Here's how the part is built. I have some questions about the finished solid (model axes, mm). Coordinates: 2 decimals unless noted, no trailing zeros. Write each loop counter-clockwise with the first axis right and the second up, starting at its lowest first coordinate (ties: lowest second). Pieces come first, ordered by that corner, then holes. Notation, with made-up numbers: (27, -0.75) -> (50, -0.75) arc R16 ccw to (50, 30.25) -> close; hole circle Ø8 at (6, 37). An arc over 180 degrees is marked (long way). Use a Markdown table: item, result. Add a question column.
Item 1: Imagine slicing it at B-B, the plane x = 0. Write out the boundary of the cut face in (y, z).
Item 2: Will these pins go through, and if not, where does the flat tip stop? pin 1 Ø4 at (x, y) = (1.5, -10.5) entering from -Z; pin 2 Ø6 at (y, z) = (3.5, 3) entering from -X; pin 3 Ø4 at (y, z) = (-18.5, 3) entering from -X; pin 4 Ø2 at (x, z) = (-4, 2.5) entering from +Y.
Item 3: Imagine slicing it at A-A, the plane z = 0. Write out the boundary of the cut face in (x, y).
Item 4: Imagine slicing it at D-D, the plane y = -25.5. Write out the boundary of the cut face in (x, z).
Item 5: Imagine slicing it at C-C, the plane y = 7. Write out the boundary of the cut face in (x, z), and give its area (3 significant figures).
Item 6: If I drill on line 1 along Z through (x, y) = (0.25, -85.5); line 2 along Z through (x, y) = (1.75, -30.5); line 3 along Y through (x, z) = (-4.25, -1.5), over which ranges is the centre line in solid material (lowest first)? Write a range as from..to.
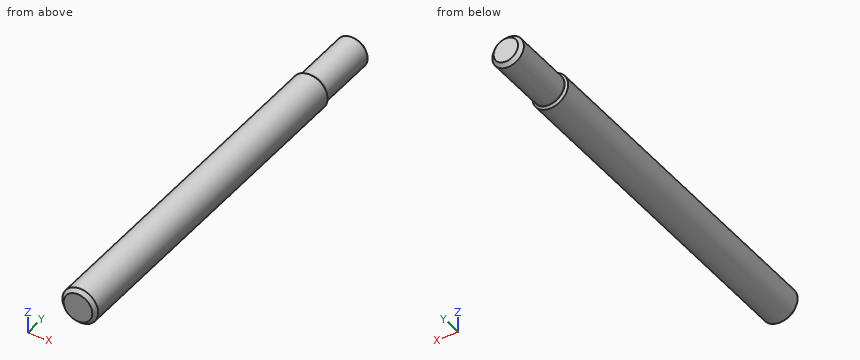
```python
from build123d import *

# Parameters (mm, degrees)
F0_R        = 5
F1_DEPTH    = 100
F2_R        = 4.4
F3_DEPTH    = 18
F4_S5_R     = 4.4
F4_T6_DEPTH = 9
F5_SIZE     = 1


# Not quite as in the source:
# - a fillet or chamfer that OpenCascade refuses, or shapes differently, is made with other operations: its cross-section is extruded or revolved along the edge and cut away or added


with BuildPart() as f1:
    # F0 (on Front) → F1 (new body)
    with BuildSketch(Plane.XZ):
        Circle(F0_R)
    extrude(amount=F1_DEPTH)

    # F2 (on face) → F3 (join)
    with BuildSketch(Plane(origin=(0, 0, 0), x_dir=(-1, 0, 0), z_dir=(0, 1, 0))):
        Circle(F2_R)
    extrude(amount=F3_DEPTH)

    # F4: chamfer of 1 on 1 edges, made by hand


with BuildPart() as f4_tool2:
    # F4_s3 → F4_t4 (revolve)
    with BuildSketch(Plane.XY):
        Polygon((5, -1), (4, 0), (5, 0), align=None)
    revolve(axis=Axis((0, 0, 0), (0, -1, 0)))

    # F4_s5 → F4_t6 (cut, symmetric)
    with BuildSketch(Plane.XZ.offset(0.5)):
        Circle(F4_S5_R)
    extrude(amount=F4_T6_DEPTH, both=True, mode=Mode.SUBTRACT)


with BuildPart() as f1_1:
    add(f1.part)

    # F4_t1: cut F4_tool2
    add(f4_tool2.part, mode=Mode.SUBTRACT)

    # F5
    f5_edges = [f1_1.edges().sort_by_distance(p)[0] for p in [
        (-5, -100, 0),
        (4.4, 18, 0),
    ]]
    chamfer(f5_edges, length=F5_SIZE)


solid = f1_1.part
```
Ans:
| question | item | result |
|---|---|---|
| 1 | outline | (-100, -4) -> (-99, -5) -> (-1, -5) -> (-0.4, -4.4) -> (17, -4.4) -> (18, -3.4) -> (18, 3.4) -> (17, 4.4) -> (-0.4, 4.4) -> (-1, 5) -> (-99, 5) -> (-100, 4) -> close |
| 2 | pin 1 | stops at z = -5 |
| 2 | pin 2 | stops at x = -4.4 |
| 2 | pin 3 | stops at x = -4.9 |
| 2 | pin 4 | stops at y = 17.68 |
| 3 | outline | (-5, -99) -> (-4, -100) -> (4, -100) -> (5, -99) -> (5, -1) -> (4.4, -0.4) -> (4.4, 17) -> (3.4, 18) -> (-3.4, 18) -> (-4.4, 17) -> (-4.4, -0.4) -> (-5, -1) -> close |
| 4 | outline | circle Ø10 at (0, 0) |
| 5 | outline | circle Ø8.8 at (0, 0) |
| 5 | area | 60.8 mm^2 |
| 6 | line 1 | z = -4.99..4.99 |
| 6 | line 2 | z = -4.68..4.68 |
| 6 | line 3 | y = -99.49..-0.51 |
